Design review of the part built by this model. Coordinates are the model's own, in mm. A direction names the side the tool comes from. Coordinates: 2 decimals unless noted, no trailing zeros. Loops run counter-clockwise (first coordinate to the right, second up) from the corner with the lowest first, then second, coordinate; pieces in that order, holes last. Notation, with made-up numbers: M -10.75,-10.5 L 29.25,-10.5 A15 ccw 29.25,3.5 Z; hole C -23,89.5 d1. An arc over 180 degrees is marked long. One line per item, written item: value.
```python
from build123d import *

# Parameters (mm, degrees)
SZKIC2_W                        = 32
SZKIC2_H                        = 67
SZKIC2_R                        = 1.375001118
SZKIC2_R_2                      = 1.375002453
SZKIC2_R_3                      = 1.374998979
SZKIC2_R_4                      = 1.375001969
DODANIE_WYCI_GNI_CIE1_DEPTH     = 1.6
SZKIC3_R                        = 2.125002003
SZKIC3_R_2                      = 2.125000412
SZKIC3_R_3                      = 2.124999361
SZKIC3_R_4                      = 2.125
DODANIE_WYCI_GNI_CIE2_DEPTH     = 4
SZKIC4_R                        = 0.85
DODANIE_WYCI_GNI_CIE3_DEPTH     = 2.3
WYTNIJ_WYCI_GNI_CIE1_DEPTH      = 75.51637404
WYTNIJ_WYCI_GNI_CIE1_DEPTH_BACK = 75.51637404
SZKIC5_W                        = 10
SZKIC5_H                        = 20
SZKIC5_H_2                      = 15
ZAOKR_GLENIE1_R                 = 1.6


with BuildPart() as part:
    # Szkic2 → Dodanie-wyciągnięcie1 (new body)
    with BuildSketch(Plane.XY):
        with Locations((16, 33.5)):
            Rectangle(SZKIC2_W, SZKIC2_H)
        with Locations((4.60000054, 4.59999621)):
            Circle(SZKIC2_R, mode=Mode.SUBTRACT)
        with Locations((27.599994617, 4.599998848)):
            Circle(SZKIC2_R_2, mode=Mode.SUBTRACT)
        with Locations((27.599997676, 62.599998714)):
            Circle(SZKIC2_R_3, mode=Mode.SUBTRACT)
        with Locations((4.599996565, 62.599994963)):
            Circle(SZKIC2_R_4, mode=Mode.SUBTRACT)
    extrude(amount=DODANIE_WYCI_GNI_CIE1_DEPTH)

    # Szkic3 → Dodanie-wyciągnięcie2 (add)
    with BuildSketch(Plane.XY.offset(1.6)):
        with Locations(Location((5.599998705, 34.699994945, 0), (0, 0, 180))):
            Circle(SZKIC3_R)
        with Locations(Location((26.599994052, 34.699996536, 0), (0, 0, 180))):
            Circle(SZKIC3_R_2)
        with Locations(Location((5.599997835, 22.199997588, 0), (0, 0, 180))):
            Circle(SZKIC3_R_3)
        with Locations(Location((26.599996674, 22.199996948, 0), (0, 0, 180))):
            Circle(SZKIC3_R_4)
    extrude(amount=DODANIE_WYCI_GNI_CIE2_DEPTH)

    # Szkic4 → Dodanie-wyciągnięcie3 (add)
    with BuildSketch(Plane.XY.offset(5.6)):
        with Locations((5.599998705, 34.699994945)):
            Circle(SZKIC4_R)
        with Locations((26.599994052, 34.699996536)):
            Circle(SZKIC4_R)
        with Locations((5.599997835, 22.199997588)):
            Circle(SZKIC4_R)
        with Locations((26.599996674, 22.199996948)):
            Circle(SZKIC4_R)
    extrude(amount=DODANIE_WYCI_GNI_CIE3_DEPTH)

    # Szkic5 → Wytnij-wyciągnięcie1 (cut, two sides: drawn at the far end of the back side and taken through both)
    with BuildSketch(Plane.XY.offset(1.6).offset(-WYTNIJ_WYCI_GNI_CIE1_DEPTH_BACK)):
        with Locations((16, 57)):
            Rectangle(SZKIC5_W, SZKIC5_H)
        with Locations((16, 7.5)):
            Rectangle(SZKIC5_W, SZKIC5_H_2)
    extrude(amount=WYTNIJ_WYCI_GNI_CIE1_DEPTH + WYTNIJ_WYCI_GNI_CIE1_DEPTH_BACK, mode=Mode.SUBTRACT)

    # Zaokrąglenie1
    zaokr_glenie1_edges = [part.edges().sort_by_distance(p)[0] for p in [
        (0, 67, 0.8),
        (21, 0, 0.8),
        (11, 15, 0.8),
        (32, 67, 0.8),
        (11, 0, 0.8),
        (21, 15, 0.8),
        (32, 0, 0.8),
        (0, 0, 0.8),
        (11, 67, 0.8),
        (21, 47, 0.8),
        (21, 67, 0.8),
        (11, 47, 0.8),
    ]]
    fillet(zaokr_glenie1_edges, radius=ZAOKR_GLENIE1_R)


solid = part.part
```
(1) We need section B-B on y = 52. State the section outline as (x, z) points, then the cut area to 3 significant figures.
Reply:
outline: M 0,0 L 11,0 L 11,1.6 L 0,1.6 Z; M 21,0 L 32,0 L 32,1.6 L 21,1.6 Z
area: 35.2 mm2
(2) We need section A-A on z = 0.75. State the section outline as (x, y) points (3 decimals), then the cut area to 3 significant figures.
Reply:
outline: M 0,1.6 A1.6 ccw 1.6,0 L 9.4,0 A1.6 ccw 11,1.6 L 11,13.4 A1.6 cw 12.6,15 L 19.4,15 A1.6 cw 21,13.4 L 21,1.6 A1.6 ccw 22.6,0 L 30.4,0 A1.6 ccw 32,1.6 L 32,65.4 A1.6 ccw 30.4,67 L 22.6,67 A1.6 ccw 21,65.4 L 21,48.6 A1.6 cw 19.4,47 L 12.6,47 A1.6 cw 11,48.6 L 11,65.4 A1.6 ccw 9.4,67 L 1.6,67 A1.6 ccw 0,65.4 Z; hole C 4.6,4.6 d2.75; hole C 4.6,62.6 d2.75; hole C 27.6,4.6 d2.75; hole C 27.6,62.6 d2.75
area: 1,770 mm2
(3) To check wall thickness, follow line 1 along Y through (x, z) = (4.6, 1) (3 decimals); line 2 along Y through (x, z) = (5.5, 3); line 3 along Z through (x, y) = (2, 20). State the ranges of each line that lie inside material, in increasing order. Write a range as [from, to].
Reply:
line 1: y = [0, 3.225], [5.975, 61.225], [63.975, 67]
line 2: y = [20.08, 24.32], [32.58, 36.82]
line 3: z = [0, 1.6]
(4) We need section D-D on z = 7. State the section outline as (x, y) points.
Reply:
outline: C 5.6,22.2 d1.7; C 5.6,34.7 d1.7; C 26.6,22.2 d1.7; C 26.6,34.7 d1.7
(5) Mouldability with a two-part tool opening along Y and no side actions: class faces 4 (the flat face through (5, 0, 1)), 5 (the cylindrical face through (20.52, 47.46, 0.81)), 6 (the flat face through (21, 7, 1)), 7 (the cylindrical face through (5.489, 35.543, 6.734)) as released by +Y, released by -Y, zero draft, split by the parting line, or undercut.
Reply:
face 4: released by -Y
face 5: released by +Y
face 6: zero draft
face 7: undercut
(6) Insertion check: pin 1 (2 mm diameter, centred on x = 4.6, y = 4.6, fed in from +Z); pin 2 (4 mm diameter, centred on x = 25, z = 4, fed in from -Y) (3 decimals); pin 3 (1.8 mm diameter, centred on x = 17, z = 0.5, fed in from +Y); pin 4 (10 mm diameter, centred on x = 5.5, y = 39, fed in from -Z). Each pin has a flat end and moves straight along its axis. Give the tip position at first contact, or say it passes through.
Reply:
pin 1: passes through
pin 2: stops at y = 20.075
pin 3: stops at y = 47
pin 4: stops at z = 0
(7) Tool access review of faces 1 (the flat face through (5, 23, 5.6)), 2 (the cylindrical face through (31.54, 0.48, 0.81)), 3 (the cylindrical face through (21.48, 0.46, 0.81)): name each direction out of +Z, -Z, +X, -X, +Y, -Y from which nothing blocks a thin tool from reaching the whole face with its end or side.
Reply:
face 1: +Z
face 2: +Z, -Z, +X, -Y
face 3: +Z, -Z, -Y
(8) We need section C-C on y = 62. State the section outline as (x, z) points.
Reply:
outline: M 0,0 L 3.36,0 L 3.36,1.6 L 0,1.6 Z; M 5.84,0 L 11,0 L 11,1.6 L 5.84,1.6 Z; M 21,0 L 26.36,0 L 26.36,1.6 L 21,1.6 Z; M 28.84,0 L 32,0 L 32,1.6 L 28.84,1.6 Z
